from build123d import *

# Parameters (mm, degrees)
F0_W     = 51
F0_H     = 51
F1_DEPTH = 30
F0_W_2   = 15
F0_H_2   = 10
F0_R     = 1.6
F0_W_3   = 10
F0_H_3   = 15
F2_DEPTH = 2
F4_DEPTH = 100
F6_DEPTH = 100


with BuildPart() as f1:
    # F0 (on Top) → F1 (new body)
    with BuildSketch(Plane.XY):
        Polygon((-7.5, 27.5), (-28.323529, 27.5), (-28.323529, 7.5), (-28.323529, -7.5), (-28.323529, -27.5), (-7.5, -27.5), (7.5, -27.5), (26.676471, -27.5), (26.676471, -7.5), (26.676471, 7.5), (26.676471, 27.5), (7.5, 27.5), align=None)
        with Locations((-0.823529, 0)):
            Rectangle(F0_W, F0_H, mode=Mode.SUBTRACT)
    extrude(amount=F1_DEPTH)

    # F0 (on Top) → F2 (join)
    with BuildSketch(Plane.XY):
        with Locations((0, 32.5)):
            Rectangle(F0_W_2, F0_H_2)
        with Locations((0, 33.877362)):
            Circle(F0_R, mode=Mode.SUBTRACT)
        with Locations((31.676471, 0)):
            Rectangle(F0_W_3, F0_H_3)
        with Locations((31.995282, 0)):
            Circle(F0_R, mode=Mode.SUBTRACT)
        with Locations((0, -32.5)):
            Rectangle(F0_W_2, F0_H_2)
        with Locations((0, -32.094341)):
            Circle(F0_R, mode=Mode.SUBTRACT)
        with Locations((-33.323529, 0)):
            Rectangle(F0_W_3, F0_H_3)
        with Locations((-33.580191, 0)):
            Circle(F0_R, mode=Mode.SUBTRACT)
    extrude(amount=F2_DEPTH)

    # F3 (on face) → F4 (cut)
    with BuildSketch(Plane.YZ.offset(26.676471)):
        Polygon((15.488846, 3.462488), (0, 27.03796), (-15.488846, 3.462488), align=None)
    extrude(amount=-F4_DEPTH, mode=Mode.SUBTRACT)

    # F5 (on face) → F6 (cut)
    with BuildSketch(Plane.XZ.offset(27.5)):
        Polygon((14.299098, 4.686049), (-1.189748, 28.261521), (-16.678594, 4.686049), align=None)
    extrude(amount=-F6_DEPTH, mode=Mode.SUBTRACT)


solid = f1.part
Could you check a few things on this model? Use its own coordinates, in mm. A direction names the side the tool comes from. Give positions to 0.01 mm unless a question says otherwise; leave off trailing zeros. Order: outer loops, then holes, each group sorted by start corner. A loop starts at its lowest first (then second) coordinate and runs counter-clockwise, first axis right, second up. Notation, with made-up numbers: (32.5, 4) - (74.5, 4) arc R17 ccw to (74.5, 29) - close; hole circle Ø10 at (86.5, -2.5). An arc over 180 degrees is marked (long way). Return JSON: item names as keys, results as strings. Group by question number.
Q1. Which directions (+Z, -Z, +X, -X, +Y, -Y) give clear straight access to the entire face, cutting with the end or side of a thin tool? Please do faces 4 (the face through (-1, 26, 4.686)), 5 (the face through (-7.5, -33, 1)), 6 (the face through (-27, 0, 3.462)), 7 (the face through (-33, 7.5, 1)), 8 (the face through (-33, 2, 2)).
Q2. Thinking about a two-plate mould opening in Y: for faces 1 (the face through (26, 0, 3.462)), 2 (the face through (7.5, 32, 1)), 3 (the face through (0, 37.5, 1)), which applies, pulls with the +Y half, pulls with the -Y half, needs draft (parallel to the pull), parting line crosses it, or undercut?
Q3. Suppose I cut it at A-A, the plane z = 9. Please give me the cut outline in (x, y).
Q4. Suppose I cut it at B-B, the plane y = 26.5. Please give me the cut outline in (x, z), and give its area (3 significant figures).
Q5. Suppose I cut it at D-D, the plane x = 0. Please give me the cut outline in (y, z).
Q6. Please list where these lines run through material, in increasing order: line 1 along Y through (x, z) = (0, 0.5); line 2 along X through (y, z) = (-14.5, 13.25); line 3 along Y through (x, z) = (-10, 26). Write a range as [from, to].
Q7. Suppose I cut it at C-C, the plane y = 10.5. Please give me the cut outline in (x, z), and give its area (3 significant figures).
Q8. Will these pins go through, and if not, where does the flat tip stop? pin 1 Ø12 at (y, z) = (-7.5, 23) entering from -X; pin 2 Ø0.6 at (x, z) = (-31, 1) entering from -Y; pin 3 Ø3.5 at (x, y) = (0, -32.09) entering from -Z; pin 4 Ø4 at (x, z) = (14.5, 3) entering from +Y.
Resolved:
{
 "1": {"face 4": "+Y, -Y", "face 5": "+Z, -Z, -X, -Y", "face 6": "+X, -X", "face 7": "+Z, -Z, -X, +Y", "face 8": "+Z, -X, +Y, -Y"},
 "2": {"face 1": "undercut", "face 2": "needs draft", "face 3": "pulls with the +Y half"},
 "3": {"outline": "(-28.32, -27.5) - (-13.84, -27.5) - (-13.84, -25.5) - (-26.32, -25.5) - (-26.32, -11.85) - (-28.32, -11.85) - close; (-28.32, 11.85) - (-26.32, 11.85) - (-26.32, 25.5) - (-13.84, 25.5) - (-13.84, 27.5) - (-28.32, 27.5) - close; (11.46, -27.5) - (26.68, -27.5) - (26.68, -11.85) - (24.68, -11.85) - (24.68, -25.5) - (11.46, -25.5) - close; (11.46, 25.5) - (24.68, 25.5) - (24.68, 11.85) - (26.68, 11.85) - (26.68, 27.5) - (11.46, 27.5) - close"},
 "4": {"outline": "(-28.32, 0) - (26.68, 0) - (26.68, 30) - (-28.32, 30) - close; hole (-16.68, 4.69) - (14.3, 4.69) - (-1.19, 28.26) - close", "area": "1,280 mm2"},
 "5": {"outline": "(-37.5, 0) - (-33.69, 0) - (-33.69, 2) - (-37.5, 2) - close; (-30.49, 0) - (-25.5, 0) - (-25.5, 4.69) - (-27.5, 4.69) - (-27.5, 2) - (-30.49, 2) - close; (-27.5, 26.45) - (-25.5, 26.45) - (-25.5, 30) - (-27.5, 30) - close; (25.5, 0) - (32.28, 0) - (32.28, 2) - (27.5, 2) - (27.5, 4.69) - (25.5, 4.69) - close; (25.5, 26.45) - (27.5, 26.45) - (27.5, 30) - (25.5, 30) - close; (35.48, 0) - (37.5, 0) - (37.5, 2) - (35.48, 2) - close"},
 "6": {"line 1": "y = [-37.5, -33.69], [-30.49, -25.5], [25.5, 32.28], [35.48, 37.5]", "line 2": "x = [-28.32, -26.32], [24.68, 26.68]", "line 3": "y = [-27.5, -25.5], [25.5, 27.5]"},
 "7": {"outline": "(-28.32, 0) - (-26.32, 0) - (-26.32, 3.46) - (-28.32, 3.46) - close; (-28.32, 11.06) - (-26.32, 11.06) - (-26.32, 30) - (-28.32, 30) - close; (24.68, 0) - (26.68, 0) - (26.68, 3.46) - (24.68, 3.46) - close; (24.68, 11.06) - (26.68, 11.06) - (26.68, 30) - (24.68, 30) - close", "area": "89.6 mm2"},
 "8": {"pin 1": "stops at x = -28.32", "pin 2": "stops at y = -7.5", "pin 3": "stops at z = 0", "pin 4": "stops at y = 27.5"}
}
